The model under review builds one solid part; all positions refer to its coordinate system, in mm. A direction names the side the tool comes from. Coordinates: 2 decimals unless noted, no trailing zeros. Order: outer loops, then holes, each group sorted by start corner. A loop starts at its lowest first (then second) coordinate and runs counter-clockwise, first axis right, second up.
from build123d import *

# Parameters (mm, degrees)
EXTRUDE_1_DEPTH     = 6
CUT_EXTRUDE_1_REACH = 24.514
SKETCH_3_R          = 1.6
FILLET_1_R          = 2


with BuildPart() as part:
    # 草图2 → 凸台-拉伸1 (new body)
    with BuildSketch(Plane(origin=(0, 0, 0), x_dir=(1, 0, 0), z_dir=(0, 1, 0))):
        Polygon((0, 0), (13.07179677, 0), (13.07179677, -4), (-6.92820323, -4), (3.07179677, 13.320508076), (6.535898385, 11.320508076), align=None)
    extrude(amount=EXTRUDE_1_DEPTH)

    # 草图3 → 切除-拉伸1 (cut, up to next)
    with BuildSketch(Plane.XY.offset(4), mode=Mode.PRIVATE) as cut_extrude_1_sk1:
        with Locations((10.07179677, 3)):
            Circle(SKETCH_3_R)
    cut_extrude_1_tool1 = extrude(cut_extrude_1_sk1.sketch, amount=-CUT_EXTRUDE_1_REACH, mode=Mode.PRIVATE) & part.part
    cut_extrude_1 = cut_extrude_1_tool1.solids().sort_by_distance((10.071797, 3, 4))[0]
    add(cut_extrude_1, mode=Mode.SUBTRACT)

    # 镜向1: 切除-拉伸1 across plane
    add(cut_extrude_1.mirror(Plane(origin=(0, 0, 0), x_dir=(-0.8660254037844399, 0, 0.4999999999999978), z_dir=(0.4999999999999983, 0, 0.8660254037844398))), mode=Mode.SUBTRACT)

    # 圆角1
    fillet_1_edges = [part.edges().sort_by_distance(p)[0] for p in [
        (0, 3, 0),
    ]]
    fillet(fillet_1_edges, radius=FILLET_1_R)


solid = part.part
(1) Wall thickness on line 1 (Z direction, x = 11.25, y = 5.4); line 2 (X direction, y = 3.65, z = 1.25); line 3 (Z direction, x = 4.75, y = 2.65): over which ranges is each line inside the solid? List them lowest first.
(2) Consider section D-D (x = 8.25). Give the boundary of the cut face in (y, z), then the cut area to 3 significant figures.
(3) Insertion check: pin 1 Ø1.5 at (y, z) = (2.5, -5.5) entering from +X; pin 2 Ø3 at (x, y) = (10.07, 3) entering from -Z; pin 3 Ø3 at (x, y) = (6.5, 4) entering from -Z; pin 4 Ø2 at (y, z) = (3, -7) entering from +X. Each pin has a flat end and moves straight along its axis. Give the tip position at first contact, or say it passes through.
(4) Consider section C-C (y = 5.15). Give the boundary of the cut face in (x, z).
(5) The part is to be moulded in two halves that separate along Y. For faces 1 (the face through (1, 0, -1)), 2 (the face through (8.8, 2.03, 2.03)), 3 (the face through (4.17, 2.29, -7.22)), 4 (the face through (3.649, 1.581, -10.376)), say which applies: +Y half, -Y half, draft (parallel to the pull), parting line (faces both ways), or undercut.
(6) Tool access review of faces 5 (the face through (8, 3, 0)), 6 (the face through (13.072, 3, 2)): name each direction out of +Z, -Z, +X, -X, +Y, -Y from which nothing blocks a thin tool from reaching the whole face with its end or side.
(7) Consider section B-B (x = 4). Give the number of separate pieces and of enclosed holes in the cut face, then the cut area to 3 significant figures.
(8) Consider section A-A (y = 3). Give the boundary of the cut face in (x, z), then the cut area to 3 significant figures.
Findings:
1. line 1: z = 0 to 4
1. line 2: x = -5.34 to 8.61, 11.53 to 13.07
1. line 3: z = -12.35 to -10.69, 0 to 4
2. outline: (0, 0) - (6, 0) - (6, 4) - (0, 4) - close
2. area: 24.0 mm2
3. pin 1: stops at x = 3.61
3. pin 2: passes through
3. pin 3: stops at z = -12.21
3. pin 4: stops at x = 4.35
4. outline: (-6.93, 4) - (3.07, -13.32) - (6.54, -11.32) - (1.73, -3) arc R2 cw to (3.46, 0) - (13.07, 0) - (13.07, 4) - close
5. face 1: -Y half
5. face 2: undercut
5. face 3: draft
5. face 4: undercut
6. face 5: +X, +Y, -Y
6. face 6: +Z, -Z, +X, +Y, -Y
7. separate pieces: 2
7. enclosed holes: 1
7. area: 49.9 mm2
8. outline: (-6.93, 4) - (0.77, -9.34) - (4.24, -7.34) - (1.73, -3) arc R2 cw to (3.46, 0) - (8.47, 0) - (8.47, 4) - close; (2.37, -12.11) - (3.07, -13.32) - (6.54, -11.32) - (5.84, -10.11) - close; (11.67, 0) - (13.07, 0) - (13.07, 4) - (11.67, 4) - close
8. area: 109 mm2
